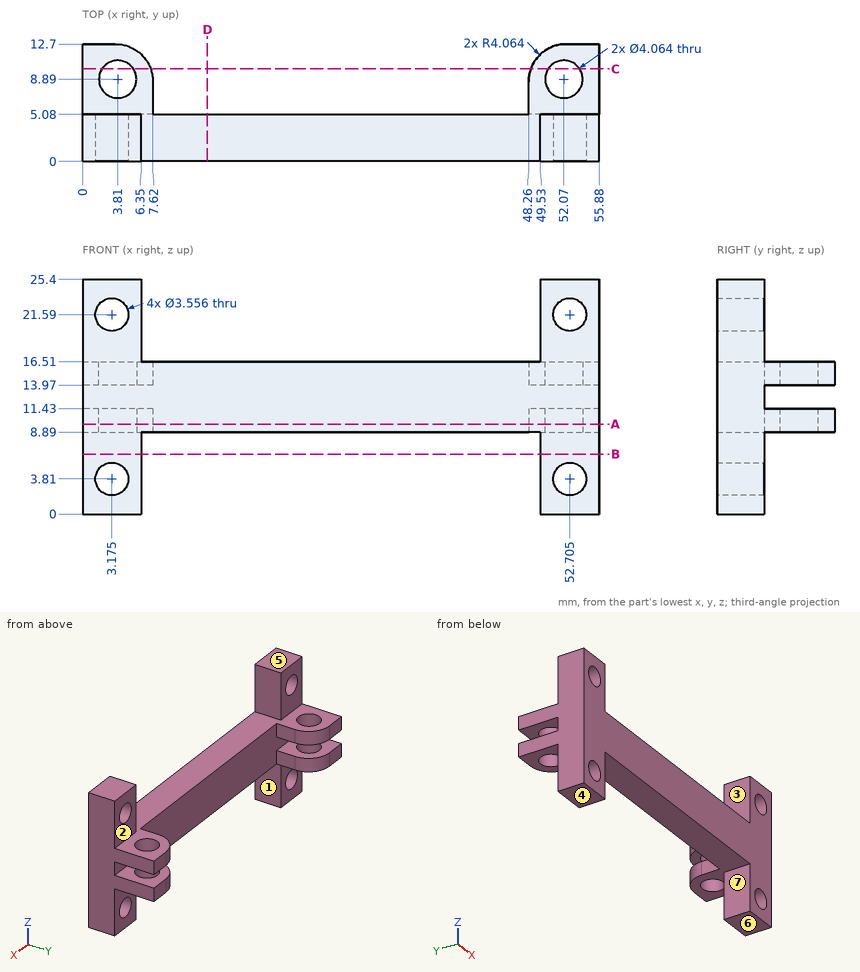
Geometry: see drawing. Coordinates: mm, zero at the bounding-box minimum. A direction names the side the tool comes from. Coordinates: 2 decimals unless noted, no trailing zeros. Order: outer loops, then holes, each group sorted by start corner. A loop starts at its lowest first (then second) coordinate and runs counter-clockwise, first axis right, second up. Notation, with made-up numbers: M -22.75,55 L 36.25,55 A22 cw 36.25,87 Z; hole C -29.5,18.5 d11. An arc over 180 degrees is marked long. Write each question's results on one line, items separated by ' | '. Start each with the question number.
1) Line query: line 1 (X direction, y = 3.55, z = 3.81); line 2 (Y direction, x = 3.81, z = 15.85); line 3 (Z direction, x = 53, y = 1.5). Output: solid intervals per line, ascending. Write a range as from..to.
2) Section query A-A (z = 9.75). Return the cut outline in (x, y), plus the area to 3 significant figures.
3) Contact query for flat-ended pins moving along their axis: pin 1 Ø4 at (x, z) = (39, 13.5) entering from +Y; pin 2 Ø4 at (x, z) = (40, 6) entering from +Y; pin 3 Ø4 at (x, y) = (3.5, 7.5) entering from +Z; pin 4 Ø4.5 at (x, y) = (3.81, 8.89) entering from -Z. Output: stop coordinate, or through.
4) Section query B-B (z = 6.5). Return the cut outline in (x, y).
5) Access query for the marked faces 1, 2, 3 and 4. Directions: +Z, -Z, +X, -X, +Y, -Y. A direction counts if a zero-diameter tool reaches every point of the face in a straight line with its end or side. Return the directions, or none.
6) Draft query along Z for the marked faces 5, 6 and 7. Return one class per face: released by +Z, released by -Z, zero draft, split by the parting line, or undercut.
7) Section query D-D (x = 13.5). Return the cut outline in (y, z).
8) Section query C-C (y = 10). Give the number of separate pieces and of enclosed holes in the cut face, plus the area to 3 significant figures.
Answers:
1) line 1: x = 0..1.4, 4.95..6.35, 49.53..50.93, 54.48..55.88 | line 2: y = 0..6.86, 10.92..12.69 | line 3: z = 0..2.06, 5.56..19.84, 23.34..25.4
2) outline: M 0,0 L 55.88,0 L 55.88,12.7 L 52.32,12.7 A4.06 ccw 48.26,8.64 L 48.26,5.08 L 7.62,5.08 L 7.62,8.64 A4.06 ccw 3.56,12.7 L 0,12.7 Z; hole C 3.81,8.89 d4.06; hole C 52.07,8.89 d4.06 | area: 367 mm^2
3) pin 1: stops at y = 5.08 | pin 2: passes through | pin 3: stops at z = 16.51 | pin 4: stops at z = 8.89
4) outline: M 0,0 L 6.35,0 L 6.35,5.08 L 0,5.08 Z; M 49.53,0 L 55.88,0 L 55.88,5.08 L 49.53,5.08 Z
5) face 1: -Z, +Y, -Y | face 2: +Z, +X, -X, +Y | face 3: +Z, +Y, -Y | face 4: -Z, +X, -X, +Y, -Y
6) face 5: released by +Z | face 6: released by -Z | face 7: zero draft
7) outline: M 0,8.89 L 5.08,8.89 L 5.08,16.51 L 0,16.51 Z
8) separate pieces: 8 | enclosed holes: 0 | area: 40.4 mm^2
